Design review of the part built by this model. Coordinates are the model's own, in mm. Face numbers are marked on the shaded views. A direction names the side the tool comes from. Coordinates: 2 decimals unless noted, no trailing zeros. Write each loop counter-clockwise with the first axis right and the second up, starting at its lowest first coordinate (ties: lowest second). Pieces come first, ordered by that corner, then holes.
Q1. Mouldability with a two-part tool opening along Y and no side actions: class the marked faces 4, 5, 6 and 7 as pulls with the +Y half, pulls with the -Y half, needs draft (parallel to the pull), parting line crosses it, or undercut.
Q2. Take a section at D-D (x = -62.25). Give the boundary of the cut face in (y, z), and give its area (3 significant figures).
Q3. Take a section at A-A (z = 20). Give the boundary of the cut face in (x, y).
Q4. For probe 1 along Y at (x, z) = (0, 6.75); probe 2 along X at (y, z) = (-27, 12.5); probe 3 along Y at (x, z) = (-15, 14.25), list the stretches that pass through material, from the lowest coordinate up.
Q5. Take a section at B-B (x = -44). Give the boundary of the cut face in (y, z).
Q6. Insertion check: pin 1 (16 mm diameter, centred on x = -53.5, y = -4.5, fed in from +Z); pin 2 (6 mm diameter, centred on x = 45, y = -4.5, fed in from -Z); pin 3 (4 mm diameter, centred on x = -62.25, y = -62.25, fed in from +Z). Each pin has a flat end and moves straight along its axis. Give the tip position at first contact, or say it passes through.
Q7. Machinability: for the marked faces 1, 2 and 3, which of the approach directions +Z, -Z, +X, -X, +Y, -Y give a long, thin tool a straight path to every point of the face, cutting with its end or side? Answer none if there is none.
Q8. Take a section at C-C (y = 48). Give the boundary of the cut face in (x, z).
```python
from build123d import *
from build123d.topology import SkipClean

# Parameters (mm, degrees)
SKICA1_W                 = 140
SKICA1_H                 = 140
P_IDAT_VYSUNUT_M1_DEPTH  = 25
SKICA2_R                 = 2.15
ODEBRAT_VYSUNUT_M1_DEPTH = 103.102889283
SKICA3_R                 = 67
SKICA3_R_2               = 17.5
ODEBRAT_VYSUNUT_M3_DEPTH = 103.102889283
P_IDAT_VYSUNUT_M2_DEPTH  = 0.5


with BuildPart() as part:
    # Skica1 → P_idat vysunut_m1 (new body)
    with BuildSketch(Plane.XY):
        Rectangle(SKICA1_W, SKICA1_H)
    extrude(amount=P_IDAT_VYSUNUT_M1_DEPTH)

    # Skica2 → Odebrat vysunut_m1 (cut, through all)
    with BuildSketch(Plane.XY.offset(25)):
        with Locations((-62.25, 62.25)):
            Circle(SKICA2_R)
        with Locations((-62.25, -62.25)):
            Circle(SKICA2_R)
        with Locations((62.25, -62.25)):
            Circle(SKICA2_R)
        with Locations((62.25, 62.25)):
            Circle(SKICA2_R)
    extrude(amount=-ODEBRAT_VYSUNUT_M1_DEPTH, mode=Mode.SUBTRACT)

    # Skica3 → Odebrat vysunut_m3 (cut, through all)
    with BuildSketch(Plane.XY.offset(25)):
        Circle(SKICA3_R)
        Circle(SKICA3_R_2, mode=Mode.SUBTRACT)
    extrude(amount=-ODEBRAT_VYSUNUT_M3_DEPTH, mode=Mode.SUBTRACT)


with BuildPart() as odebrat_vysunut_m3_piece_1:
    # of the separate pieces the step leaves, piece 1, a body of its own (odebrat_vysunut_m3_pieces)
    add(part.part.solids().sort_by_distance((-70, 70, 0))[0])



with BuildPart() as odebrat_vysunut_m3_piece_2:
    # of the separate pieces the step leaves, piece 2, a body of its own (odebrat_vysunut_m3_pieces)
    add(part.part.solids().sort_by_distance((17.5, 0, 0))[0])


with BuildPart() as odebrat_vysunut_m3_piece_1_1:
    with SkipClean():  # the faces are left unmerged after this step: merging them gives an invalid solid
        add(odebrat_vysunut_m3_piece_1.part)

        add(odebrat_vysunut_m3_piece_2.part)  # P_idat vysunut_m2 merges Odebrat vysunut_m3 piece 2
        # Skica4 → P_idat vysunut_m2 (add, symmetric)
        with BuildSketch(Plane(origin=(0, 0, 12.5), x_dir=(-1, 0, 0), z_dir=(0, 0, -1))):
            with BuildLine():
                Line((-10, 66.2495283), (-10, 14.361406616))
                ThreePointArc((-10, 14.361406616), (-12.374368671, 12.374368671), (-14.361406616, 10))
                Line((-14.361406616, 10), (-66.2495283, 10))
                ThreePointArc((-66.2495283, 10), (-67, 0), (-66.2495283, -10))
                Line((-66.2495283, -10), (-14.361406616, -10))
                ThreePointArc((-14.361406616, -10), (-12.374368671, -12.374368671), (-10, -14.361406616))
                Line((-10, -14.361406616), (-10, -66.2495283))
                ThreePointArc((-10, -66.2495283), (0, -67), (10, -66.2495283))
                Line((10, -66.2495283), (10, -14.361406616))
                ThreePointArc((10, -14.361406616), (12.374368671, -12.374368671), (14.361406616, -10))
                Line((14.361406616, -10), (66.2495283, -10))
                ThreePointArc((66.2495283, -10), (67, 0), (66.2495283, 10))
                Line((66.2495283, 10), (14.361406616, 10))
                ThreePointArc((14.361406616, 10), (12.374368671, 12.374368671), (10, 14.361406616))
                Line((10, 14.361406616), (10, 66.2495283))
                ThreePointArc((10, 66.2495283), (0, 67), (-10, 66.2495283))
            make_face()
        extrude(amount=P_IDAT_VYSUNUT_M2_DEPTH, both=True)


solid = odebrat_vysunut_m3_piece_1_1.part
```
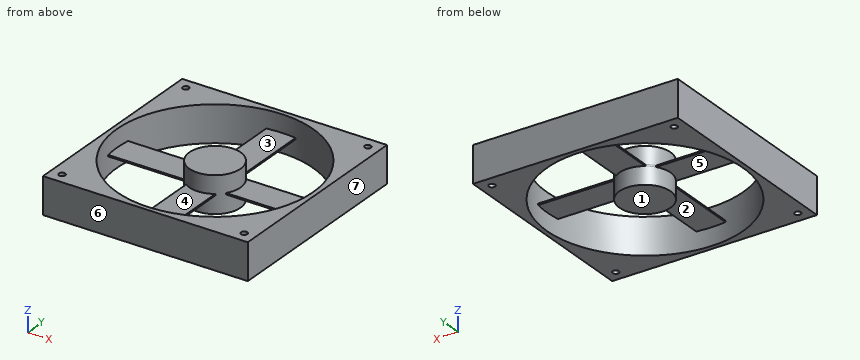
Response:
1. face 4: undercut
1. face 5: undercut
1. face 6: pulls with the -Y half
1. face 7: needs draft
2. outline: (-70, 0) - (-64.4, 0) - (-64.4, 25) - (-70, 25) - close; (-60.1, 0) - (-24.78, 0) - (-24.78, 25) - (-60.1, 25) - close; (-10, 12) - (10, 12) - (10, 13) - (-10, 13) - close; (24.78, 0) - (60.1, 0) - (60.1, 25) - (24.78, 25) - close; (64.4, 0) - (70, 0) - (70, 25) - (64.4, 25) - close
2. area: 2,070 mm2
3. outline: (-70, -70) - (70, -70) - (70, 70) - (-70, 70) - close; circle Ø35 at (0, 0); hole circle Ø134 at (0, 0); hole circle Ø4.3 at (-62.25, -62.25); hole circle Ø4.3 at (-62.25, 62.25); hole circle Ø4.3 at (62.25, -62.25); hole circle Ø4.3 at (62.25, 62.25)
4. probe 1: y = -70 to -67, -17.5 to 17.5, 67 to 70
4. probe 2: x = -70 to -61.32, -10 to 10, 61.32 to 70
4. probe 3: y = -70 to -65.3, -9.01 to 9.01, 65.3 to 70
5. outline: (-70, 0) - (-50.53, 0) - (-50.53, 25) - (-70, 25) - close; (-10, 12) - (10, 12) - (10, 13) - (-10, 13) - close; (50.53, 0) - (70, 0) - (70, 25) - (50.53, 25) - close
6. pin 1: stops at z = 13
6. pin 2: stops at z = 12
6. pin 3: passes through
7. face 1: -Z, +X, -X, +Y, -Y
7. face 2: -Z
7. face 3: +Z
8. outline: (-70, 0) - (-46.74, 0) - (-46.74, 25) - (-70, 25) - close; (-10, 12) - (10, 12) - (10, 13) - (-10, 13) - close; (46.74, 0) - (70, 0) - (70, 25) - (46.74, 25) - close
